from build123d import *

# Parameters (mm, degrees)
BOSS_EXTRUDE1_DEPTH = 2
SKETCH2_W           = 95.5
SKETCH2_H           = 2
BOSS_EXTRUDE2_DEPTH = 10
SKETCH3_R           = 3
CUT_EXTRUDE1_DEPTH  = 34
SKETCH4_W           = 46.5
SKETCH4_H           = 1
BOSS_EXTRUDE3_DEPTH = 3


with BuildPart() as part:
    # Sketch1 → Boss-Extrude1 (new body)
    with BuildSketch(Plane.XY):
        Polygon((-2.998624877, 17.747280284), (-0.498624877, 17.747280284), (-0.498624877, -11.252719716), (46.001375123, -11.252719716), (46.001375123, 21.747280284), (-49.498624877, 21.747280284), (-49.498624877, -11.252719716), (-2.998624877, -11.252719716), align=None)
    extrude(amount=BOSS_EXTRUDE1_DEPTH)

    # Sketch2 → Boss-Extrude2 (add)
    with BuildSketch(Plane.XY.offset(2)):
        with Locations((-1.748624877, 20.747280284)):
            Rectangle(SKETCH2_W, SKETCH2_H)
    extrude(amount=BOSS_EXTRUDE2_DEPTH)

    # Sketch3 → Cut-Extrude1 (cut, through all)
    with BuildSketch(Plane(origin=(0, 21.747280284, 0), x_dir=(1, 0, 0), z_dir=(0, 1, 0))):
        with Locations((-45.248624877, -6)):
            Circle(SKETCH3_R)
        with Locations((-7.248624877, -6)):
            Circle(SKETCH3_R)
        with Locations((3.751375123, -6)):
            Circle(SKETCH3_R)
        with Locations((41.751375123, -6)):
            Circle(SKETCH3_R)
    extrude(amount=-CUT_EXTRUDE1_DEPTH, mode=Mode.SUBTRACT)

    # Sketch4 → Boss-Extrude3 (add)
    with BuildSketch(Plane(origin=(0, 0, 0), x_dir=(-1, 0, 0), z_dir=(0, 0, -1))):
        with Locations((-22.751375123, -10.752719716)):
            Rectangle(SKETCH4_W, SKETCH4_H)
        with Locations((26.248624877, -10.752719716)):
            Rectangle(SKETCH4_W, SKETCH4_H)
    extrude(amount=BOSS_EXTRUDE3_DEPTH)


solid = part.part
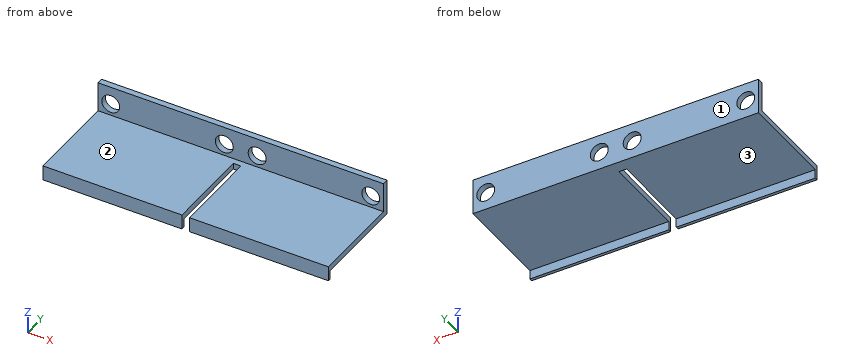
Read the model definition and answer for the solid it produces. Units are mm, in the model's axes. Face numbers are marked on the shaded views. A direction names the side the tool comes from. Coordinates: 2 decimals unless noted, no trailing zeros. Order: outer loops, then holes, each group sorted by start corner. A loop starts at its lowest first (then second) coordinate and runs counter-clockwise, first axis right, second up. Notation, with made-up numbers: M 13,76 L 34,76 A22 ccw 34,84 Z; hole C 24.25,12 d5. An arc over 180 degrees is marked long. Put each result on its own line as item: value. Start each with the question number.
Item 1: For the marked faces 1, 2 and 3, determine the directions among +Z, -Z, +X, -X, +Y, -Y from which every point of the face is accessible in a straight line to the end or side of a thin tool.
Item 2: Consider probe 1 along X at (y, z) = (20.95, 6); probe 2 along X at (y, z) = (2, 1.75); probe 3 along Z at (x, y) = (8, -9.5). Determine where each line is inside the solid, lowest interval first. Write a range as [from, to].
Item 3: Given pin 1 Ø1.5 at (y, z) = (-1.5, -1.5) entering from +X (3 decimals); pin 2 Ø12 at (x, y) = (-18, 4.5) entering from -Z; pin 3 Ø15.5 at (x, y) = (16.5, 2.5) entering from +Z; pin 4 Ø5 at (x, z) = (-20.5, 5.5) entering from -Y, each flat-ended and moving along its own axis, determine where each tip first touches the part or whether it passes through.
Item 4: Section C-C, the plane y = -4 is taken. Determine the outline of the cut face in (x, z), plus the area to 3 significant figures.
Item 5: Section D-D, the plane x = -8.5 is taken. Determine the outline of the cut face in (y, z).
Item 6: Section A-A, the plane z = 6 is taken. Determine the outline of the cut face in (x, y).
Item 7: Section B-B, the plane x = 26.5 is taken. Determine the outline of the cut face in (y, z), plus the area to 3 significant figures.
Computed:
1. face 1: +Z, -Z, +X, -X, +Y
1. face 2: +Z, +X, -X, -Y
1. face 3: -Z, +X, -X, +Y
2. probe 1: x = [-49.5, -48.25], [-42.25, -10.25], [-4.25, 0.75], [6.75, 38.75], [44.75, 46]
2. probe 2: x = [-49.5, -3], [-0.5, 46]
2. probe 3: z = [0, 2]
3. pin 1: passes through
3. pin 2: stops at z = 0
3. pin 3: stops at z = 2
3. pin 4: stops at y = 19.75
4. outline: M -49.5,0 L -3,0 L -3,2 L -49.5,2 Z; M -0.5,0 L 46,0 L 46,2 L -0.5,2 Z
4. area: 186 mm2
5. outline: M -11.25,-3 L -10.25,-3 L -10.25,0 L 21.75,0 L 21.75,3.27 L 19.75,3.27 L 19.75,2 L -11.25,2 Z; M 19.75,8.73 L 21.75,8.73 L 21.75,12 L 19.75,12 Z
6. outline: M -49.5,19.75 L -48.25,19.75 L -48.25,21.75 L -49.5,21.75 Z; M -42.25,19.75 L -10.25,19.75 L -10.25,21.75 L -42.25,21.75 Z; M -4.25,19.75 L 0.75,19.75 L 0.75,21.75 L -4.25,21.75 Z; M 6.75,19.75 L 38.75,19.75 L 38.75,21.75 L 6.75,21.75 Z; M 44.75,19.75 L 46,19.75 L 46,21.75 L 44.75,21.75 Z
7. outline: M -11.25,-3 L -10.25,-3 L -10.25,0 L 21.75,0 L 21.75,12 L 19.75,12 L 19.75,2 L -11.25,2 Z
7. area: 89.0 mm2
